```python
from build123d import *

# Parameters (mm, degrees)
F0_R     = 2.1
F1_DEPTH = 3.5
F2_R     = 4.99999
F3_R     = 2.1
F4_DEPTH = 4


# Not quite as in the source:
# - a fillet or chamfer is up to 0.001 mm smaller than in the source, because OpenCascade refuses the exact size
# - ends of sketch curves that miss each other by under 0.0002 mm in the source are joined


with BuildPart() as f1:
    # F0 (on Top) → F1 (new body)
    with BuildSketch(Plane.XY):
        Polygon((1.4820488868, -12.5), (5, -12.5), (5, 12.5), (-5, 12.5), (-5, -12.5), (-1.4866787242, -12.5), (-1.4866787242, 3.6), (1.4820488868, 3.6), align=None)
        with Locations((0, 8.5)):
            Circle(F0_R, mode=Mode.SUBTRACT)
    extrude(amount=F1_DEPTH)

    # F2 (radius 5 in the source; OpenCascade refuses exactly that, so slightly less here)
    f2_edges = [f1.edges().sort_by_distance(p)[0] for p in [
        (-5, 12.5, 1.75),
        (5, 12.5, 1.75),
    ]]
    fillet(f2_edges, radius=F2_R)

    # F3 (on face) → F4 (join)
    with BuildSketch(Plane.XY.offset(3.5)):
        with BuildLine():
            Line((-5, 3.6241896451), (0, 3.6241896451))
            Line((0, 3.6241896451), (5, 3.6241896451))
            Line((5, 3.6241896451), (5, 7.50001))
            ThreePointArc((5, 7.50001), (3.5355368349, 11.0355368349), (1e-05, 12.5))
            ThreePointArc((1e-05, 12.5), (-3.5355368349, 11.0355368349), (-5, 7.50001))
            Line((-5, 7.50001), (-5, 3.6241896451))
        make_face()
        with Locations((0, 8.5)):
            Circle(F3_R, mode=Mode.SUBTRACT)
    extrude(amount=F4_DEPTH)


solid = f1.part
```
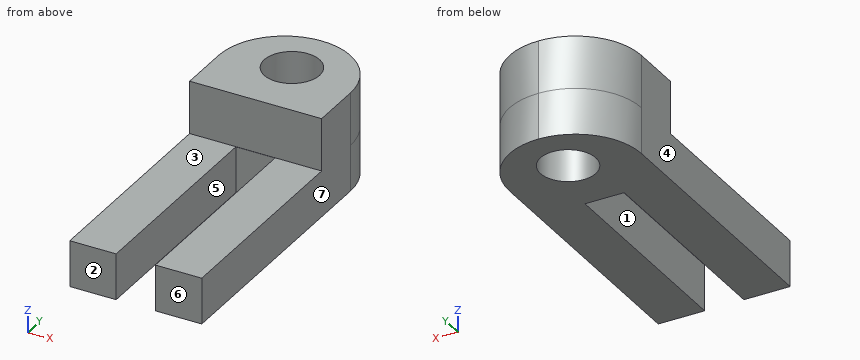
For this review, take the finished solid that the model builds, in its own axes (mm). Face numbers are marked on the shaded views. A direction names the side the tool comes from. Round coordinates to 2 decimals unless told otherwise and drop trailing zeros. Write each loop counter-clockwise with the first axis right and the second up, starting at its lowest first coordinate (ties: lowest second). Pieces come first, ordered by that corner, then holes. Notation, with made-up numbers: (-29, 5) - (19, 5) arc R30 ccw to (19, 32) - close; hole circle Ø3 at (-6.75, 88). An arc over 180 degrees is marked (long way). Use CSV: the item, a comma, the result in double quotes.
1) Add section D-D on x = 4.25. Write out the cut boundary in (y, z).
Conclusion:
outline,"(-12.5, 0) - (10.13, 0) - (10.13, 7.5) - (3.62, 7.5) - (3.62, 3.5) - (-12.5, 3.5) - close"
2) Clearance check with flat-ended pins moving along their axes: pin 1 Ø4 at (y, z) = (10, 1.5) entering from +X; pin 2 Ø1 at (x, z) = (1, 3.5) entering from +Y; pin 3 Ø1 at (x, z) = (-2, 5) entering from -Y. State where each tip first meets the part, or that it passes through.
Conclusion:
pin 1,"stops at x = 4.97"
pin 2,"stops at y = 12.47"
pin 3,"stops at y = 3.62"
3) Wall thickness on line 1 along Y through (x, z) = (0, 3.75); line 2 along Z through (x, y) = (3.5, 1); line 3 along Y through (x, z) = (2.5, 6): over which ranges is each line inside the solid? List them lowest first. Write a range as from..to.
Conclusion:
line 1,"y = 3.62..6.4, 10.6..12.5"
line 2,"z = 0..3.5"
line 3,"y = 3.62..11.83"
4) The part is to be moulded in two halves that separate along X. For the marked faces 4, 5, 6 and 7, say which applies: pulls with the +X half, pulls with the -X half, needs draft (parallel to the pull), parting line crosses it, or undercut.
Conclusion:
face 4,"pulls with the -X half"
face 5,"undercut"
face 6,"needs draft"
face 7,"pulls with the +X half"
5) For the marked faces 1, 2 and 3, list the 3-axis set-ups (+Z, -Z, +X, -X, +Y, -Y) from which the entire face can be reached by the end or side of a thin tool; tool diameter is ignored.
Conclusion:
face 1,"+Z, -Z, -Y"
face 2,"+Z, -Z, +X, -X, -Y"
face 3,"+Z, +X, -X, -Y"
6) Add section B-B on y = 8.5. Write out the cut boundary in (x, z), and give its area (3 significant figures).
Conclusion:
outline,"(-4.9, 0) - (-2.1, 0) - (-2.1, 7.5) - (-4.9, 7.5) - close; (2.1, 0) - (4.9, 0) - (4.9, 7.5) - (2.1, 7.5) - close"
area,"42.0 mm^2"
